CAD build for the part. Positions are in the model's coordinates, mm. Face numbers are marked on the shaded views. A direction names the side the tool comes from. Coordinates: 2 decimals unless noted, no trailing zeros. Loops run counter-clockwise (first coordinate to the right, second up) from the corner with the lowest first, then second, coordinate; pieces in that order, holes last. Notation, with made-up numbers: (6, 41.5) -> (56, 41.5) arc R32 ccw to (56, 72.5) -> close; hole circle Ø7 at (55, 44.25). An arc over 180 degrees is marked (long way). Write each question's results on one line, items separated by ' | '.
```python
from build123d import *

# Parameters (mm, degrees)
BOX001_W     = 60
BOX001_H     = 30
BOX001_DEPTH = 32
BOX_W        = 33.5
BOX_H        = 40
BOX_DEPTH    = 48


with BuildPart() as box001:
    # Box001 → Box001 (new body)
    with BuildSketch(Plane(origin=(-14, 5, 8), x_dir=(1, 0, 0), z_dir=(0, 0, 1))):
        with Locations((30, 15)):
            Rectangle(BOX001_W, BOX001_H)
    extrude(amount=BOX001_DEPTH)


with BuildPart() as obj1:
    # Box → Box (new body)
    with BuildSketch(Plane.XY):
        with Locations((16.75, 20)):
            Rectangle(BOX_W, BOX_H)
    extrude(amount=BOX_DEPTH)

    # Fusion: union Box001
    add(box001.part)


solid = obj1.part
```
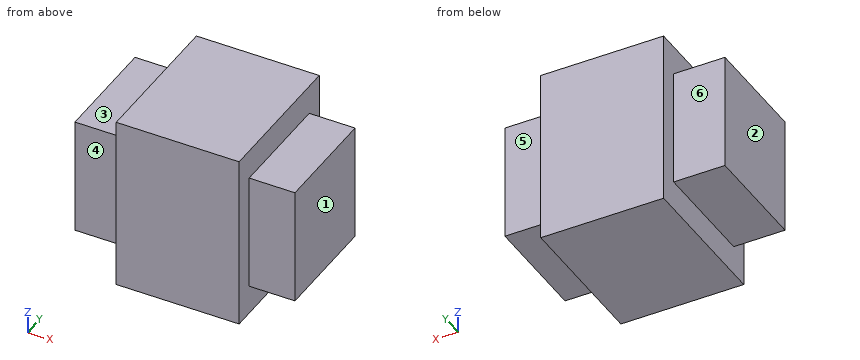
Q1. Wall check: L1, parallel to Z at x = -2.5, y = 21.5; L2, parallel to X at y = 3, z = 40. Give the ranges that are in metal, low to high. Write a range as from..to.
Results are:
L1: 8..40 | L2: 0..33.5
Q2. Drop flat-ended pins along their axis: pin 1 (1 mm diameter, centred on x = -2.5, z = 26.5, fed in from +Y); pin 2 (10 mm diameter, centred on x = 43, y = 20, fed in from -Z); pin 3 (10 mm diameter, centred on x = 41.5, z = 27, fed in from -Y). Give the stop position or say it passes through.
Results are:
pin 1: y = 35 | pin 2: z = 8 | pin 3: y = 5
Q3. Which spindle directions (+Z, -Z, +X, -X, +Y, -Y) get a long thin tool onto all of the face, cutting with end or side? Do the marked faces 4, 5 and 6. Say none if no direction does.
Results are:
face 4: +Z, -Z, -X, -Y | face 5: +Z, -Z, +X, +Y | face 6: +Z, -Z, -X, +Y
Q4. Cut at B-B on z = 26.5. Write the cut outline in (x, y), and give its area (4 significant figures).
Results are:
outline: (-14, 5) -> (0, 5) -> (0, 0) -> (33.5, 0) -> (33.5, 5) -> (46, 5) -> (46, 35) -> (33.5, 35) -> (33.5, 40) -> (0, 40) -> (0, 35) -> (-14, 35) -> close | area: 2,135 mm^2
Q5. Cut at A-A on y = 16.5. Write the cut outline in (x, z), and give its area (3 significant figures).
Results are:
outline: (-14, 8) -> (0, 8) -> (0, 0) -> (33.5, 0) -> (33.5, 8) -> (46, 8) -> (46, 40) -> (33.5, 40) -> (33.5, 48) -> (0, 48) -> (0, 40) -> (-14, 40) -> close | area: 2,460 mm^2
Q6. Pull direction X, two halves, no side cores. Call the marked faces 1, 2 and 3: +X half, -X half, draft (parallel to the pull), parting line (faces both ways), or undercut.
Results are:
face 1: +X half | face 2: -X half | face 3: draft
Q7. Cut at C-C on x = 39.5. Write the cut outline in (y, z).
Results are:
outline: (5, 8) -> (35, 8) -> (35, 40) -> (5, 40) -> close
Q8. Cut at D-D on z = 3. Write the cut outline in (x, y), and give its area (3 significant figures).
Results are:
outline: (0, 0) -> (33.5, 0) -> (33.5, 40) -> (0, 40) -> close | area: 1,340 mm^2
